Here's how the part is built. I have some questions about the finished solid (model axes, mm). Face numbers are marked on the shaded views. A direction names the side the tool comes from. Round coordinates to 2 decimals unless told otherwise and drop trailing zeros. Order: outer loops, then holes, each group sorted by start corner. A loop starts at its lowest first (then second) coordinate and runs counter-clockwise, first axis right, second up. Notation, with made-up numbers: (-18.5, -4.5) -> (10.5, -4.5) arc R21 ccw to (10.5, 14.5) -> close; hole circle Ø6 at (1.5, 78). An arc over 180 degrees is marked (long way). One line per item, written item: value.
```python
from build123d import *

# Parameters (mm, degrees)
SKETCH_1_W          = 78.62
SKETCH_1_H          = 50
EXTRUDE_1_DEPTH     = 12
SKETCH_3_W          = 50.02416134
SKETCH_3_H          = 10
CUT_EXTRUDE_1_DEPTH = 94.942026804
FILLET_3_R          = 20
FILLET_4_R          = 20
SKETCH_5_R          = 2.5
CUT_EXTRUDE_3_DEPTH = 20
SKETCH_6_W          = 50.02416134
SKETCH_6_H          = 80
EXTRUDE_2_DEPTH     = 12
FILLET_5_R          = 10
SKETCH_7_R          = 2.5
CUT_EXTRUDE_4_DEPTH = 30


with BuildPart() as part:
    # Эскиз1 → Бобышка-Вытянуть1 (new body)
    with BuildSketch(Plane.XY):
        with Locations((39.31, 25)):
            Rectangle(SKETCH_1_W, SKETCH_1_H)
    extrude(amount=EXTRUDE_1_DEPTH)

    # Эскиз3 → Вырез-Вытянуть1 (cut, through all)
    with BuildSketch(Plane.XY.offset(12)):
        Polygon((19.858926821, 50), (78.62, 28.952063791), (78.62, 50), align=None)
        with Locations((53.60791933, 5)):
            Rectangle(SKETCH_3_W, SKETCH_3_H)
    extrude(amount=-CUT_EXTRUDE_1_DEPTH, mode=Mode.SUBTRACT)

    # Скругление3
    fillet_3_edges = [part.edges().sort_by_distance(p)[0] for p in [
        (78.62, 28.952063791, 6),
    ]]
    fillet(fillet_3_edges, radius=FILLET_3_R)

    # Скругление4
    fillet_4_edges = [part.edges().sort_by_distance(p)[0] for p in [
        (19.858926821, 50, 6),
    ]]
    fillet(fillet_4_edges, radius=FILLET_4_R)

    # Эскиз5 → Вырез-Вытянуть3 (cut)
    with BuildSketch(Plane.ZY):
        with Locations(Location((6, 7, 0), (0, 0, 270))):
            Circle(SKETCH_5_R)
        with Locations(Location((6, 41, 0), (0, 0, 270))):
            Circle(SKETCH_5_R)
    extrude(amount=-CUT_EXTRUDE_3_DEPTH, mode=Mode.SUBTRACT)

    # Эскиз6 → Бобышка-Вытянуть2 (add)
    with BuildSketch(Plane.XY.offset(12)):
        with Locations((53.60791933, -30)):
            Rectangle(SKETCH_6_W, SKETCH_6_H)
    extrude(amount=-EXTRUDE_2_DEPTH)

    # Скругление5
    fillet_5_edges = [part.edges().sort_by_distance(p)[0] for p in [
        (28.59583866, 0, 6),
    ]]
    fillet(fillet_5_edges, radius=FILLET_5_R)

    # Эскиз7 → Вырез-Вытянуть4 (cut)
    with BuildSketch(Plane.XZ.offset(70)):
        with Locations(Location((38.59583866, 6, 0), (0, 0, 270))):
            Circle(SKETCH_7_R)
        with Locations(Location((68.59583866, 6, 0), (0, 0, 270))):
            Circle(SKETCH_7_R)
    extrude(amount=-CUT_EXTRUDE_4_DEPTH, mode=Mode.SUBTRACT)


solid = part.part
```
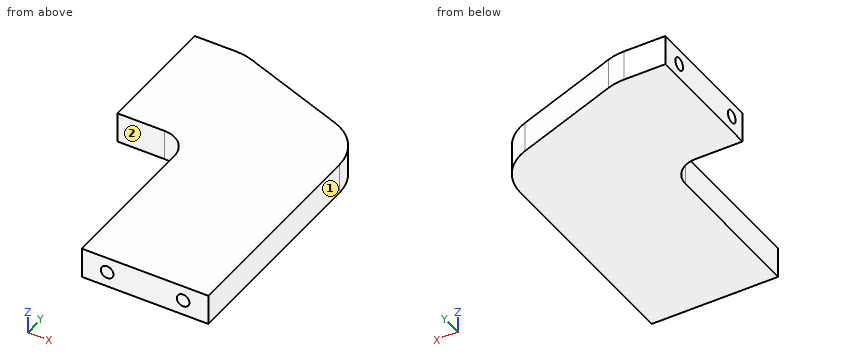
Q1. I want a section at A-A on x = 11. Write out the boundary of the cut face in (y, z), then the cut area to 3 significant figures.
Answers:
outline: (0, 0) -> (50, 0) -> (50, 12) -> (0, 12) -> close; hole circle Ø5 at (7, 6); hole circle Ø5 at (41, 6)
area: 561 mm2
Q2. I want a section at B-B on y = 7. Write out the boundary of the cut face in (x, z).
Answers:
outline: (0, 0) -> (78.62, 0) -> (78.62, 12) -> (0, 12) -> (0, 8.5) -> (20, 8.5) -> (20, 3.5) -> (0, 3.5) -> close
Q3. I want a section at C-C on z = 6. Write out the boundary of the cut face in (x, y).
Answers:
outline: (0, 0) -> (18.6, 0) arc R10 cw to (28.6, -10) -> (28.6, -70) -> (36.1, -70) -> (36.1, -40) -> (41.1, -40) -> (41.1, -70) -> (66.1, -70) -> (66.1, -40) -> (71.1, -40) -> (71.1, -70) -> (78.62, -70) -> (78.62, 14.87) arc R20 ccw to (65.36, 33.7) -> (23.13, 48.83) arc R20 ccw to (16.39, 50) -> (0, 50) -> (0, 43.5) -> (20, 43.5) -> (20, 38.5) -> (0, 38.5) -> (0, 9.5) -> (20, 9.5) -> (20, 4.5) -> (0, 4.5) -> close
Q4. I want a section at D-D on y = -46.5. Write out the boundary of the cut face in (x, z).
Answers:
outline: (28.6, 0) -> (78.62, 0) -> (78.62, 12) -> (28.6, 12) -> close; hole circle Ø5 at (38.6, 6); hole circle Ø5 at (68.6, 6)
Q5. Which directions (+Z, -Z, +X, -X, +Y, -Y) give clear straight access to the entire face, cutting with the end or side of a thin tool? Please do the marked faces 1 and 2.
Answers:
face 1: +Z, -Z, +X, +Y, -Y
face 2: +Z, -Z, -X, -Y
Q6. I need wall thicknesses on line 1 along X through (y, z) = (-49.5, 6); line 2 along Z through (x, y) = (11, 41); line 3 along X through (y, z) = (-58, 7.75). Which ranges of each line are inside material? Lowest first, please.
Answers:
line 1: 28.6 to 36.1, 41.1 to 66.1, 71.1 to 78.62
line 2: 0 to 3.5, 8.5 to 12
line 3: 28.6 to 36.81, 40.38 to 66.81, 70.38 to 78.62
Q7. For P1, Ø5.5, axis at y = 42, z = 5.5, coming from the -X side; P2, Ø6.5, axis at x = 38.6, z = 6, coming from the +Y side; P3, Ø2.5, axis at y = 7.5, z = 6.5, coming from the -X side; P4, Ø3.5, axis at x = 6.5, z = 8.5, coming from the -Y side, each with a flat end and sliding along its axis, tell me the tip position at first contact or that it passes through.
Answers:
P1: x = 0
P2: y = 44.45
P3: x = 20
P4: y = 0
